```python
from build123d import *

# Parameters (mm, degrees)
BOSS_EXTRUDE1_DEPTH = 1.6


with BuildPart() as part:
    # Sketch1 → Boss-Extrude1 (new body)
    with BuildSketch(Plane(origin=(0, 0, 0), x_dir=(1, 0, 0), z_dir=(0, 1, 0))):
        with BuildLine():
            Line((-23.247910864, 15.801225627), (54.752089136, 15.801225627))
            Line((54.752089136, 15.801225627), (54.752089136, 11.841225627))
            Line((54.752089136, 11.841225627), (46.552089136, 11.841225627))
            Line((46.552089136, 11.841225627), (46.552089136, -4.038774373))
            Line((46.552089136, -4.038774373), (50.022089136, -4.038774373))
            Line((50.022089136, -4.038774373), (50.022089136, -11.338774373))
            Line((50.022089136, -11.338774373), (43.742089136, -11.338774373))
            Line((43.742089136, -11.338774373), (43.742089136, -1.438774373))
            Line((43.742089136, -1.438774373), (30.692089136, -1.438774373))
            Line((30.692089136, -1.438774373), (30.692089136, -9.998774373))
            Line((30.692089136, -9.998774373), (25.362089136, -9.998774373))
            Line((25.362089136, -9.998774373), (25.362089136, -1.438774373))
            Line((25.362089136, -1.438774373), (12.312089136, -1.438774373))
            Line((12.312089136, -1.438774373), (12.312089136, -9.998774373))
            Line((12.312089136, -9.998774373), (6.982089136, -9.998774373))
            Line((6.982089136, -9.998774373), (6.982089136, -1.438774373))
            Line((6.982089136, -1.438774373), (-6.067910864, -1.438774373))
            Line((-6.067910864, -1.438774373), (-6.067910864, -9.998774373))
            Line((-6.067910864, -9.998774373), (-11.397910864, -9.998774373))
            Line((-11.397910864, -9.998774373), (-11.397910864, -1.438774373))
            Line((-11.397910864, -1.438774373), (-24.447910864, -1.438774373))
            Line((-24.447910864, -1.438774373), (-24.447910864, -9.998774373))
            add(Edge.make_bspline(
                [(-24.447910864, -9.998774373), (-29.341121858, -6.518559079), (-29.797910864, 11.691225627)],
                knots=[0, 0, 0, 1, 1, 1], degree=2))
            Line((-29.797910864, 11.691225627), (-23.247910864, 11.691225627))
            Line((-23.247910864, 11.691225627), (-23.247910864, 15.801225627))
        make_face()
    extrude(amount=BOSS_EXTRUDE1_DEPTH)


solid = part.part
```
Check sheet for the modelled part. Datum: model origin and axes. Units: mm. A direction names the side the tool comes from. Coordinates: 2 decimals unless noted, no trailing zeros. Order: outer loops, then holes, each group sorted by start corner. A loop starts at its lowest first (then second) coordinate and runs counter-clockwise, first axis right, second up. Notation, with made-up numbers: M 59,42 L 103,42 A20 ccw 103,71 Z; hole C -24,5.5 d5. An arc over 180 degrees is marked long. One line per question, with ' | ' between items. Start each with the question number.
Item 1: Sectioned sample at A-A on x = 22. Record the cut outline in (y, z).
Item 2: Gauge pin test, flat ends, axial feed: P1, Ø0.5, axis at y = 1, z = -2.5, coming from the +X side; P2, Ø0.8, axis at x = 51, y = 0.5, coming from the +Z side; P3, Ø0.5, axis at y = 1, z = 7, coming from the -X side. Record the tip position at first contact, or that the pin passes through.
Item 3: Sectioned sample at B-B on z = -14. Record the cut outline in (x, y), and give its area (3 significant figures).
Item 4: Mould release check, pull along Z, two halves, no side actions. Record for faces 1 (the flat face through (43.742, 1, 6)), 2 (the flat face through (46.552, 1, -4)), 3 (the flat face through (10, 1, 9.999)), 4 (the flat face through (51, 1, -11.841)): pulls with the +Z half, pulls with the -Z half, needs draft (parallel to the pull), parting line crosses it, or undercut.
Item 5: Access from +Z, -Z, +X, -X, +Y, -Y to the whole of each face (thin tool, end or side, straight path). Record for faces 5 (the flat face through (50.022, 1, 8)), 6 (the flat face through (6.982, 1, 6)), 7 (the flat face through (-23.248, 1, -14)).
Item 6: Material ranges on line 1 (Z direction, x = 48.5, y = 0.1); line 2 (X direction, y = 0.9, z = 3); line 3 (X direction, y = 0.1, z = 1.75), recorded low to high.
Item 7: Sectioned sample at C-C on z = 5.25. Count the separate pieces of the cut face and the enclosed holes in it, and give its area (3 significant figures).
Answer below:
1) outline: M 0,-15.8 L 1.6,-15.8 L 1.6,1.44 L 0,1.44 Z
2) P1: stops at x = 46.55 | P2: stops at z = -11.84 | P3: stops at x = -26.91
3) outline: M -23.25,0 L 54.75,0 L 54.75,1.6 L -23.25,1.6 Z | area: 125 mm^2
4) face 1: needs draft | face 2: undercut | face 3: pulls with the +Z half | face 4: undercut
5) face 5: +Z, +X, +Y, -Y | face 6: +Z, +Y, -Y | face 7: -Z, -X, +Y, -Y
6) line 1: z = -15.8 to -11.84, 4.04 to 11.34 | line 2: x = -28.19 to -24.45, -11.4 to -6.07, 6.98 to 12.31, 25.36 to 30.69, 43.74 to 46.55 | line 3: x = -28.48 to -24.45, -11.4 to -6.07, 6.98 to 12.31, 25.36 to 30.69, 43.74 to 46.55
7) separate pieces: 5 | enclosed holes: 0 | area: 40.5 mm^2
